Part print with two shaded views. Sizes in mm from the minimum x, y, z corner. A direction names the side the tool comes from. Round coordinates to 2 decimals unless told otherwise and drop trailing zeros. Write each loop counter-clockwise with the first axis right and the second up, starting at its lowest first coordinate (ties: lowest second). Pieces come first, ordered by that corner, then holes. Notation, with made-up numbers: (-27, -26) - (-4, -26) arc R10 ccw to (-4, -21) - close; hole circle Ø3 at (69.5, 86). An arc over 180 degrees is marked (long way). Answer as a JSON object with one key per item and string values. Group by question number.
Item 1: Flat gauge pins, fed straight in: pin 1 (0.6 mm diameter, centred on x = 14.5, z = 2, fed in from +Y); pin 2 (20 mm diameter, centred on x = 15.5, y = 33, fed in from +Z); pin 3 (1 mm diameter, centred on y = 81, z = 2, fed in from -X). Where does each tip first touch, or does it go through?
Item 2: Slice it at B-B, the plane y = 116.8. List the corners of the cut face in (x, z).
Item 3: Slice it at A-A, the plane z = 5.5. List the corners of the cut face in (x, y), then the cut area to 3 significant figures.
Item 4: Slice it at D-D, the plane y = 60.5. List the corners of the cut face in (x, z), then the cut area to 3 significant figures.
Item 5: Slice it at C-C, the plane x = 12. List the corners of the cut face in (y, z), then the cut area to 3 significant figures.
Item 6: Probe line 1 (Y direction, x = 35.5, z = 1.5); line 2 (Y direction, x = 4.5, z = 3.5); line 3 (X direction, y = 116.8, z = 2). List the from-to ranges inside material, lowest first. Write a range as from..to.
Item 7: Which spindle directions (+Z, -Z, +X, -X, +Y, -Y) get a long thin tool onto all of the face, cutting with end or side? Do the marked faces 1 and 2. Say none if no direction does.
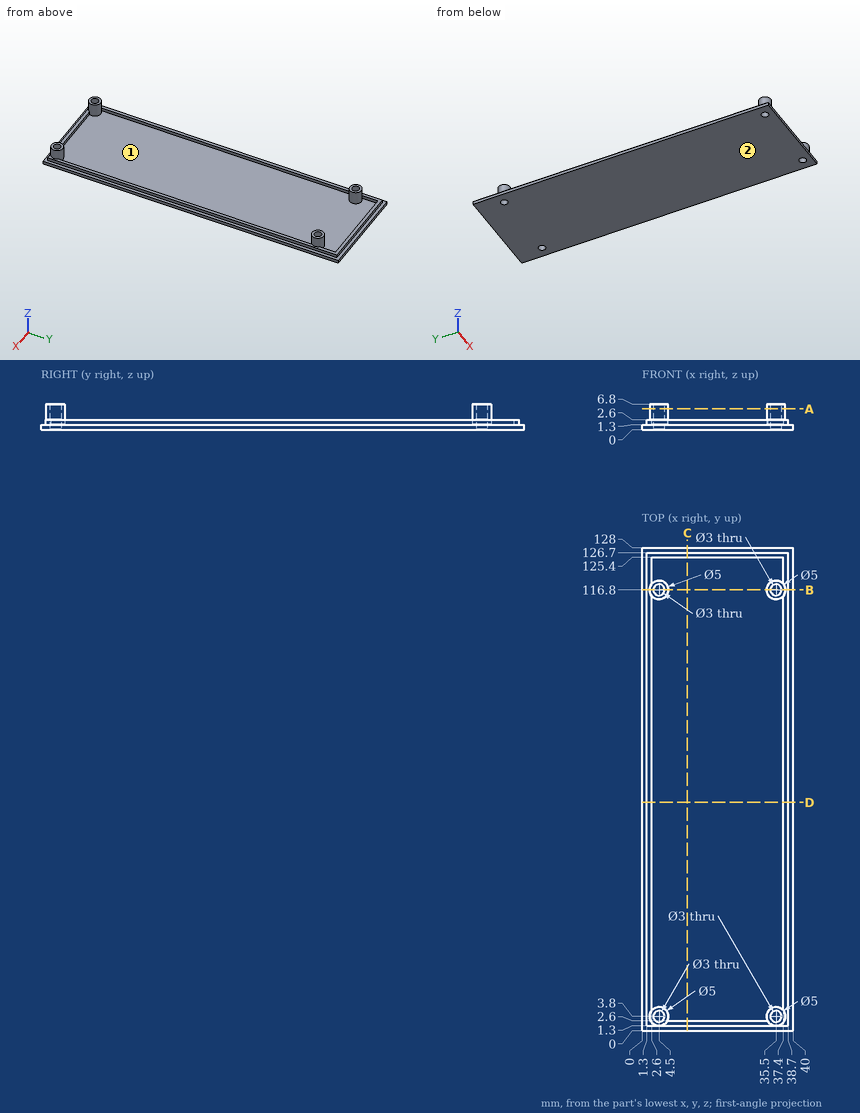
Geometry says:
{
 "1": {"pin 1": "stops at y = 126.7", "pin 2": "stops at z = 1.3", "pin 3": "stops at x = 1.3"},
 "2": {"outline": "(0, 0) - (3, 0) - (3, 6.8) - (2, 6.8) - (2, 2.6) - (1.3, 2.6) - (1.3, 1.3) - (0, 1.3) - close; (6, 0) - (34, 0) - (34, 6.8) - (33, 6.8) - (33, 1.3) - (7, 1.3) - (7, 6.8) - (6, 6.8) - close; (37, 0) - (40, 0) - (40, 1.3) - (38.7, 1.3) - (38.7, 2.6) - (38, 2.6) - (38, 6.8) - (37, 6.8) - close"},
 "3": {"outline": "circle Ø5 at (4.5, 3.8); circle Ø5 at (4.5, 116.8); circle Ø5 at (35.5, 3.8); circle Ø5 at (35.5, 116.8); hole circle Ø3 at (4.5, 3.8); hole circle Ø3 at (4.5, 116.8); hole circle Ø3 at (35.5, 3.8); hole circle Ø3 at (35.5, 116.8)", "area": "50.3 mm^2"},
 "4": {"outline": "(0, 0) - (40, 0) - (40, 1.3) - (38.7, 1.3) - (38.7, 2.6) - (37.4, 2.6) - (37.4, 1.3) - (2.6, 1.3) - (2.6, 2.6) - (1.3, 2.6) - (1.3, 1.3) - (0, 1.3) - close", "area": "55.4 mm^2"},
 "5": {"outline": "(0, 0) - (128, 0) - (128, 1.3) - (126.7, 1.3) - (126.7, 2.6) - (125.4, 2.6) - (125.4, 1.3) - (2.6, 1.3) - (2.6, 2.6) - (1.3, 2.6) - (1.3, 1.3) - (0, 1.3) - close", "area": "170 mm^2"},
 "6": {"line 1": "y = 1.3..2.3, 5.3..6.3, 114.3..115.3, 118.3..119.3, 125.4..126.7", "line 2": "y = 1.3..2.3, 5.3..6.3, 114.3..115.3, 118.3..119.3", "line 3": "x = 1.3..3, 6..7, 33..34, 37..38.7"},
 "7": {"face 1": "+Z", "face 2": "-Z, +X, -X, +Y, -Y"}
}
